from build123d import *

# Parameters (mm, degrees)
SKETCH1_W               = 20
SKETCH1_H               = 10
BOSS_EXTRUDE1_DEPTH     = 10
SKETCH3_W               = 20
SKETCH3_H               = 5
BOSS_EXTRUDE2_DEPTH     = 20
FILLET1_R               = 10
BOSS_EXTRUDE3_DEPTH     = 20
CUT_EXTRUDE1_DEPTH      = 56.733742024
CUT_EXTRUDE1_DEPTH_BACK = 56.733742024
SKETCH5_R               = 2.75
CHAMFER1_SIZE           = 10
SKETCH6_W               = 20
SKETCH6_H               = 5
BOSS_EXTRUDE4_DEPTH     = 25
FILLET2_R               = 10
CUT_EXTRUDE2_DEPTH      = 76
CUT_EXTRUDE2_DEPTH_BACK = 15
SKETCH7_R               = 2.75
CHAMFER3_SIZE           = 5
CUT_EXTRUDE3_DEPTH      = 2.5


# Some blends are built 0.0001 mm under size
with BuildPart() as part:
    # Sketch1 → Boss-Extrude1 (new body)
    with BuildSketch(Plane.XY):
        Rectangle(SKETCH1_W, SKETCH1_H)
    extrude(amount=BOSS_EXTRUDE1_DEPTH)

    # Sketch3 → Boss-Extrude2 (add)
    with BuildSketch(Plane(origin=(0, 0, 0), x_dir=(-1, 0, 0), z_dir=(0, 0, -1))):
        Rectangle(SKETCH3_W, SKETCH3_H)
    extrude(amount=BOSS_EXTRUDE2_DEPTH)

    # Fillet1
    fillet1_edges = [part.edges().sort_by_distance(p)[0] for p in [
        (-10, 0, -20),
        (10, 0, -20),
    ]]
    fillet(fillet1_edges, radius=FILLET1_R - 0.0001)  # a hair under: the kernel refuses the full size

    # Sketch4 → Boss-Extrude3 (add)
    with BuildSketch(Plane.ZY.offset(10)):
        Polygon((20, -5), (20, 15), (50, 15), (50, 25), (10, 25), (10, -5), align=None)
    extrude(amount=-BOSS_EXTRUDE3_DEPTH)

    # Sketch5 → Cut-Extrude1 (cut, two sides: drawn at the far end of the back side and taken through both)
    with BuildSketch(Plane(origin=(0, 2.5, 0), x_dir=(1, 0, 0), z_dir=(0, 1, 0)).offset(-CUT_EXTRUDE1_DEPTH_BACK)):
        with Locations(Location((0, 10, 0), (0, 0, 270))):
            Circle(SKETCH5_R)
    extrude(amount=CUT_EXTRUDE1_DEPTH + CUT_EXTRUDE1_DEPTH_BACK, mode=Mode.SUBTRACT)

    # Chamfer1
    # the kernel refuses this chamfer: 10 mm, written as the material it takes off along each edge
    with BuildSketch(Plane(origin=(35.71682988, 5, 0), x_dir=(0, -0.9996219169112968, -0.027495876610586372), z_dir=(-1, 0, 0))) as chamfer1_piece_1_section:
        Polygon((CHAMFER1_SIZE * 0.999621916911, CHAMFER1_SIZE * 0.0274958766106), (-CHAMFER1_SIZE * 0.0274958766106, CHAMFER1_SIZE * 0.999621916911), (0, 0), align=None)
    chamfer1_piece_1 = extrude(amount=71.433659759, mode=Mode.PRIVATE)
    chamfer1_piece_1 = split(chamfer1_piece_1, bisect_by=Plane(origin=(0, -2.5, 0.578931494), z_dir=(0, -1, 0)), keep=Keep.TOP, mode=Mode.PRIVATE)
    add(chamfer1_piece_1, mode=Mode.SUBTRACT)
    with BuildSketch(Plane(origin=(35.71682988, 5, 0), x_dir=(0, -0.9996219169112968, -0.027495876610586372), z_dir=(-1, 0, 0))) as chamfer1_piece_2_section:
        Polygon((CHAMFER1_SIZE * 0.999621916911, CHAMFER1_SIZE * 0.0274958766106), (-CHAMFER1_SIZE * 0.0274958766106, CHAMFER1_SIZE * 0.999621916911), (0, 0), align=None)
    chamfer1_piece_2 = extrude(amount=71.433659759, mode=Mode.PRIVATE)
    chamfer1_piece_2 = split(chamfer1_piece_2, bisect_by=Plane(origin=(0, 2.5, 4.466280687), z_dir=(0, 1, 0)), keep=Keep.TOP, mode=Mode.PRIVATE)
    chamfer1_piece_2 = split(chamfer1_piece_2, bisect_by=Plane(origin=(0, 3.939233337, 10), z_dir=(0, 0, -1)), keep=Keep.TOP, mode=Mode.PRIVATE)
    add(chamfer1_piece_2, mode=Mode.SUBTRACT)
    with BuildSketch(Plane(origin=(-35.71682988, -5, 0), x_dir=(0, -0.027495876610586403, 0.9996219169112968), z_dir=(1, 0, 0))) as chamfer1_piece_3_section:
        Polygon((CHAMFER1_SIZE * 0.999621916911, -CHAMFER1_SIZE * 0.0274958766106), (-CHAMFER1_SIZE * 0.0274958766106, -CHAMFER1_SIZE * 0.999621916911), (0, 0), align=None)
    chamfer1_piece_3 = extrude(amount=71.433659759, mode=Mode.PRIVATE)
    chamfer1_piece_3 = split(chamfer1_piece_3, bisect_by=Plane(origin=(0, -2.5, 4.487529346), z_dir=(0, -1, 0)), keep=Keep.TOP, mode=Mode.PRIVATE)
    add(chamfer1_piece_3, mode=Mode.SUBTRACT)
    with BuildSketch(Plane(origin=(-35.71682988, -5, 0), x_dir=(0, -0.027495876610586403, 0.9996219169112968), z_dir=(1, 0, 0))) as chamfer1_piece_4_section:
        Polygon((CHAMFER1_SIZE * 0.999621916911, -CHAMFER1_SIZE * 0.0274958766106), (-CHAMFER1_SIZE * 0.0274958766106, -CHAMFER1_SIZE * 0.999621916911), (0, 0), align=None)
    chamfer1_piece_4 = extrude(amount=71.433659759, mode=Mode.PRIVATE)
    chamfer1_piece_4 = split(chamfer1_piece_4, bisect_by=Plane(origin=(0, 2.5, 0.578931494), z_dir=(0, 1, 0)), keep=Keep.TOP, mode=Mode.PRIVATE)
    add(chamfer1_piece_4, mode=Mode.SUBTRACT)

    # Sketch6 → Boss-Extrude4 (add)
    with BuildSketch(Plane.XZ.offset(-15)):
        with Locations((0, 37.5)):
            Rectangle(SKETCH6_W, SKETCH6_H)
        with Locations((0, 47.5)):
            Rectangle(SKETCH6_W, SKETCH6_H)
    extrude(amount=BOSS_EXTRUDE4_DEPTH)

    # Fillet2
    fillet2_edges = [part.edges().sort_by_distance(p)[0] for p in [
        (10, -10, 37.5),
        (-10, -10, 37.5),
        (-10, -10, 47.5),
        (10, -10, 47.5),
    ]]
    fillet(fillet2_edges, radius=FILLET2_R - 0.0001)  # a hair under: the kernel refuses the full size

    # Sketch7 → Cut-Extrude2 (cut, two sides: drawn at the far end of the back side and taken through both)
    with BuildSketch(Plane.XY.offset(50).offset(-CUT_EXTRUDE2_DEPTH_BACK)):
        Circle(SKETCH7_R)
    extrude(amount=CUT_EXTRUDE2_DEPTH + CUT_EXTRUDE2_DEPTH_BACK, mode=Mode.SUBTRACT)

    # Chamfer3
    chamfer3_edges = [part.edges().sort_by_distance(p)[0] for p in [
        (0, 15, 35),
        (0, 25, 10),
        (0, 25, 50),
        (0, 15, 20),
        (0, -5, 20),
    ]]
    chamfer(chamfer3_edges, length=CHAMFER3_SIZE)

    # Sketch8 → Cut-Extrude3 (cut)
    with BuildSketch(Plane.XY.offset(50)):
        Polygon((4.731883381, -1.301004613), (3.492644735, 3.447428909), (-1.239238646, 4.748433522), (-4.731883381, 1.301004613), (-3.492644735, -3.447428909), (1.239238646, -4.748433522), align=None)
    extrude(amount=-CUT_EXTRUDE3_DEPTH, mode=Mode.SUBTRACT)


solid = part.part
Can you work these out from the model? Positions are in its coordinate system, mm. A direction names the side the tool comes from. Give positions to 0.01 mm unless a question says otherwise; leave off trailing zeros. Loops run counter-clockwise (first coordinate to the right, second up) from the corner with the lowest first, then second, coordinate; pieces in that order, holes last. Notation, with made-up numbers: M 47.25,55.25 L 97.25,55.25 A14 cw 97.25,73.25 Z; hole C -29,83 d4. An arc over 180 degrees is marked long. One line per item, written item: value. Start each with the question number.
1) Thinking about a two-plate mould opening in Y: for faces 5 (the face through (-0.596, -2.685, 46.232)), 6 (the face through (0, 5, 45)), 7 (the face through (0, 12, 22)), which applies, +Y half, -Y half, draft (parallel to the pull), parting line (faces both ways), or undercut?
2) If we section it at D-D, the plane x = 7.5: Write out the boundary of the cut face in (y, z), and give its area (3 significant figures).
3) If we section it at A-A, the plane y = 14: Write out the boundary of the cut face in (x, z).
4) On a 3-axis mill with a long thin cutter (end or side, diameter ignored), from which of +Z, -Z, +X, -X, +Y, -Y can I reach the whole of each face in a straight line? I mean faces 1 (the face through (0, -2.5, -6)), 2 (the face through (0, 5, 40)), 3 (the face through (0, 2.5, -6)), 4 (the face through (1.16, 4.09, 48.77)). Say none if no direction works.
5) If we section it at C-C, the plane y = -7: Write out the boundary of the cut face in (x, z), and give its area (3 significant figures).
6) I'm going to push flat-ended pins straight in: pin 1 (5.5 mm diameter, centred on x = -1, z = 13.5, fed in from -Y); pin 2 (7 mm diameter, centred on x = 0, y = 0, fed in from +Z); pin 3 (5.5 mm diameter, centred on x = 3, z = 27, fed in from -Y). Where does each tip first touch, or does it pass through?
7) If we section it at B-B, the plane z = -9: Write out the boundary of the cut face in (x, y).
8) If I drill on line 1 (Z direction, x = -2.5, y = 8.5); line 2 (X direction, y = 0, z = 46); line 3 (Y direction, x = 0, z = 37.5), over which ranges is the centre line in solid material (lowest first)? Write a range as [from, to].
Completed:
1. face 5: undercut
1. face 6: draft
1. face 7: -Y half
2. outline: M -6.61,35 L 10,35 L 15,30 L 15,25 L 10,20 L 0,20 L -5,15 L -5,10 L -2.5,7.5 L -2.5,-16.61 L 2.5,-16.61 L 2.5,7.5 L 5,10 L 20,10 L 25,15 L 25,45 L 20,50 L -6.61,50 L -6.61,45 L 15,45 L 15,40 L -6.61,40 Z
2. area: 943 mm^2
3. outline: M -10,10 L 10,10 L 10,24 L -10,24 Z; M -10,31 L 10,31 L 10,40 L -10,40 Z; M -10,45 L 10,45 L 10,50 L -10,50 Z
4. face 1: -Z, +X, -X, -Y
4. face 2: +X, -X, -Y
4. face 3: -Z, +X, -X, +Y
4. face 4: +Z
5. outline: M -7.14,35 L 7.14,35 L 7.14,40 L -7.14,40 Z; M -7.14,45 L 7.14,45 L 7.14,50 L -7.14,50 Z
5. area: 143 mm^2
6. pin 1: stops at y = -5
6. pin 2: stops at z = 47.5
6. pin 3: stops at y = 14.25
7. outline: M -10,-2.5 L -2.56,-2.5 L -2.56,2.5 L -10,2.5 Z; M 2.56,-2.5 L 10,-2.5 L 10,2.5 L 2.56,2.5 Z
8. line 1: z = [10, 20], [35, 40], [45, 50]
8. line 2: x = [-10, -2.75], [2.75, 10]
8. line 3: y = [-10, -2.75], [2.75, 25]
